Work out the finished part from the listing and answer in its coordinate system (mm). A direction names the side the tool comes from. Coordinates: 2 decimals unless noted, no trailing zeros. Write item = value, one per line. Start each with the question number.
Q1. Flat-ended cylindrical pins translate along their axes: pin 1 (3 mm diameter, centred on x = 41, y = -9, fed in from +Z); pin 2 (2 mm diameter, centred on x = 55.5, y = -10.5, fed in from +Z); pin 3 (1 mm diameter, centred on y = -10.5, z = 26, fed in from -X); pin 4 (8 mm diameter, centred on y = -18.5, z = 20.5, fed in from -X). Find the tip coordinate at first contact, or state that the pin passes through.
Q2. Which of the six approach directions +Z, -Z, +X, -X, +Y, -Y give full straight-line access (tool end or side, diameter ignored) to faces 1 (the cylindrical face through (46.12, -19, 70.07)), 2 (the cylindrical face through (46, -2, 1)), 3 (the cylindrical face through (46.75, -19, 1.43)), 4 (the cylindrical face through (58.655, -10.324, 72.47)), 5 (the cylindrical face through (62.71, -1.43, 76.99))?
Q3. For a pull along X with two mould halves and no side action, classify faces 6 (the cylindrical face through (29.835, -18.996, 77.085)), 7 (the flat face through (46, 0, 42)), 8 (the cylindrical face through (2.923, -3.082, 41.236)) as +X half, -X half, draft (parallel to the pull), parting line (faces both ways), or undercut.
Q4. Straight lines are drawn through the part: L1, parallel to Z at x = 41.5, y = -6; L2, parallel to Z at x = 77, y = -17; L3, parallel to X at y = -2.25, z = 28.5. For each, find the intervals that lie inside material, in ascending order. Write a range as from..to.
```python
from build123d import *

# Parameters (mm, degrees)
F1_DEPTH = 20.5
F2_R     = 10.24999
F3_F1_R  = 5
F3_F2_R  = 5
F5_DEPTH = 10


# Not quite as in the source:
# - a fillet or chamfer is up to 0.001 mm smaller than in the source, because OpenCascade refuses the exact size


with BuildPart() as f1:
    # F0 (on Front) → F1 (new body)
    with BuildSketch(Plane.XZ):
        Polygon((0, 83.5), (0, 0), (46.25, 0), (46.25, 71.5), (33.2, 71.5), (29.2, 83.5), align=None)
        Polygon((46.25, 71.5), (46.25, 0), (92.5, 0), (92.5, 83.5), (63.3, 83.5), (59.3, 71.5), align=None)
    extrude(amount=F1_DEPTH)

    # F2 (radius 10.25 in the source; OpenCascade refuses exactly that, so slightly less here)
    f2_edges = [f1.edges().sort_by_distance(p)[0] for p in [
        (0, -20.5, 41.75),
        (0, 0, 41.75),
        (92.5, -20.5, 41.75),
        (92.5, 0, 41.75),
    ]]
    fillet(f2_edges, radius=F2_R)

    # F3: fillet of radius 5 on 24 edges, made by hand

    # F3_f1
    f3_f1_edges = [f1.edges().sort_by_distance(p)[0] for p in [
        (59.3, -10.25, 71.5),
        (33.2, -10.25, 71.5),
    ]]
    fillet(f3_f1_edges, radius=F3_F1_R)

    # F3_f2
    f3_f2_edges = [f1.edges().sort_by_distance(p)[0] for p in [
        (92.5, -10.25, 83.5),
        (89.4978474361, -3.0021525639, 83.5),
        (89.4978474361, -17.4978474361, 83.5),
        (72.775005, 0, 83.5),
        (72.775005, -20.5, 83.5),
        (63.3, -10.25, 83.5),
        (0, -10.25, 83.5),
        (3.0021525639, -3.0021525639, 83.5),
        (3.0021525639, -17.4978474361, 83.5),
        (19.724995, 0, 83.5),
        (19.724995, -20.5, 83.5),
        (29.2, -10.25, 83.5),
        (0, -10.25, 0),
        (3.0021525639, -3.0021525639, 0),
        (3.0021525639, -17.4978474361, 0),
        (46.25, 0, 0),
        (46.25, -20.5, 0),
        (89.4978474361, -3.0021525639, 0),
        (89.4978474361, -17.4978474361, 0),
        (92.5, -10.25, 0),
        (46.25, 0, 71.5),
        (46.25, -20.5, 71.5),
        (58.619755323, -20.5, 72.4437890741),
        (33.880244677, -20.5, 72.4437890741),
        (58.619755323, 0, 72.4437890741),
        (33.880244677, 0, 72.4437890741),
    ]]
    fillet(f3_f2_edges, radius=F3_F2_R)

    # F4 (on face) → F5 (join)
    with BuildSketch(Plane.XY.offset(71.5)):
        with BuildLine():
            ThreePointArc((46.25, -15.5), (49.9623106012, -13.9623106012), (51.5, -10.25))
            ThreePointArc((51.5, -10.25), (49.9623106012, -6.5376893988), (46.25, -5))
            ThreePointArc((46.25, -5), (41, -10.25), (46.25, -15.5))
        make_face()
    extrude(amount=F5_DEPTH)


solid = f1.part
```
Model answer:
q1.pin_1 = 81.5
q1.pin_2 = 71.57
q1.pin_3 = 0
q1.pin_4 = 0.92
q2.face_1 = +Z, -Y
q2.face_2 = -Z, +X, -X, +Y
q2.face_3 = -Z, +X, -X, -Y
q2.face_4 = +Z, +Y, -Y
q2.face_5 = +Z, +Y
q3.face_6 = undercut
q3.face_7 = draft
q3.face_8 = -X half
q4.L1 = 0..71.5
q4.L2 = 0.23..83.27
q4.L3 = 3.84..88.66
